from build123d import *

# Parameters (mm, degrees)
SKETCH1_W                    = 286
SKETCH1_H                    = 27
SKETCH1_R                    = 2
BOSS_EXTRUDE1_DEPTH          = 3
EDGE_FLANGE3_STRIP_W         = 13
EDGE_FLANGE3_STRIP_H         = 3
EDGE_FLANGE3_STRIP_CUT_DEPTH = 286
EDGE_FLANGE3_DEPTH           = 286


# Sheet-metal steps are written as plain solids
with BuildPart() as part:
    # Sketch1 → Boss-Extrude1 (new body)
    with BuildSketch(Plane(origin=(0, 0, 0), x_dir=(1, 0, 0), z_dir=(0, 1, 0))):
        with Locations((-143, 13.5)):
            Rectangle(SKETCH1_W, SKETCH1_H)
        with Locations(Location((-278, 21.5, 0), (0, 0, 270))):
            Circle(SKETCH1_R, mode=Mode.SUBTRACT)
        with Locations(Location((-278, 5.5, 0), (0, 0, 270))):
            Circle(SKETCH1_R, mode=Mode.SUBTRACT)
        with Locations(Location((-8, 21.5, 0), (0, 0, 90))):
            Circle(SKETCH1_R, mode=Mode.SUBTRACT)
        with Locations(Location((-8, 5.5, 0), (0, 0, 90))):
            Circle(SKETCH1_R, mode=Mode.SUBTRACT)
    extrude(amount=BOSS_EXTRUDE1_DEPTH)

    # Edge-Flange3 strip (across the edge) → Edge-Flange3 strip cut (cut)
    with BuildSketch(Plane(origin=(0, 3, -27), x_dir=(0, 0, 1), z_dir=(-1, 0, 0))):
        with Locations((-6, -1.5)):
            Rectangle(EDGE_FLANGE3_STRIP_W, EDGE_FLANGE3_STRIP_H)
    extrude(amount=EDGE_FLANGE3_STRIP_CUT_DEPTH, mode=Mode.SUBTRACT)

    # Edge-Flange3 section (across the edge) → Edge-Flange3 (add)
    with BuildSketch(Plane(origin=(0, 3, -27), x_dir=(0, 0, 1), z_dir=(-1, 0, 0))):
        with BuildLine():
            Line((-3, 0.5), (-3, 10))
            Line((-3, 10), (0, 10))
            Line((0, 10), (0, 0.5))
            ThreePointArc((0, 0.5), (0.146446609, 0.146446609), (0.5, 0))
            Line((0.5, 0), (0.5, -3))
            ThreePointArc((0.5, -3), (-1.974873734, -1.974873734), (-3, 0.5))
        make_face()
    extrude(amount=EDGE_FLANGE3_DEPTH)


solid = part.part
Here's how the part is built. I have some questions about the finished solid (model axes, mm). A direction names the side the tool comes from. Coordinates: 2 decimals unless noted, no trailing zeros. Order: outer loops, then holes, each group sorted by start corner. A loop starts at its lowest first (then second) coordinate and runs counter-clockwise, first axis right, second up. Notation, with made-up numbers: (79, 70) -> (116, 70) arc R16 cw to (116, 95) -> close; hole circle Ø9 at (-8.5, 6.25). An arc over 180 degrees is marked (long way). Answer in a Markdown table with one row per item.
(1) I want a section at C-C on z = -12. List the corners of the cut face in (x, y) for me, then the cut area to 3 significant figures.
Answer key:
| item | result |
|---|---|
| outline | (-286, 0) -> (0, 0) -> (0, 3) -> (-286, 3) -> close |
| area | 858 mm^2 |
(2) On a 3-axis mill with a long thin cutter (end or side, diameter ignored), from which of +Z, -Z, +X, -X, +Y, -Y can I reach the whole of each face in a straight line? I mean faces 1 (the face through (-145, 0, -13)), 2 (the face through (-141, 8, -27)). Say none if no direction works.
Answer key:
| item | result |
|---|---|
| face 1 | +Z, -Z, +X, -X, -Y |
| face 2 | +Z, +X, -X, +Y |
(3) I want a section at B-B on y = 7.75. List the corners of the cut face in (x, z) for me, then the cut area to 3 significant figures.
Answer key:
| item | result |
|---|---|
| outline | (-286, -30) -> (0, -30) -> (0, -27) -> (-286, -27) -> close |
| area | 858 mm^2 |
(4) Please list where these lines run through material, in increasing order: probe 1 along Z at (x, y) = (-8, 1.75); probe 2 along Z at (x, y) = (-8, 1.6); probe 3 along Y at (x, z) = (-261.5, -23.5).
Answer key:
| item | result |
|---|---|
| probe 1 | -29.53 to -23.5, -19.5 to -7.5, -3.5 to 0 |
| probe 2 | -29.44 to -23.5, -19.5 to -7.5, -3.5 to 0 |
| probe 3 | 0 to 3 |
(5) I want a section at A-A on x = -130. List the corners of the cut face in (y, z) for me, then the cut area to 3 significant figures.
Answer key:
| item | result |
|---|---|
| outline | (0, -26.5) arc R3.5 ccw to (3.5, -30) -> (13, -30) -> (13, -27) -> (3.5, -27) arc R0.5 cw to (3, -26.5) -> (3, 0) -> (0, 0) -> close |
| area | 117 mm^2 |
(6) Will these pins go through, and if not, where does the flat tip stop? pin 1 Ø3 at (x, z) = (-110.5, -7) entering from -Y; pin 2 Ø7.5 at (x, y) = (-129.5, 8.5) entering from +Z; pin 3 Ø2 at (x, z) = (-156, -24) entering from +Y.
Answer key:
| item | result |
|---|---|
| pin 1 | y = 0 |
| pin 2 | z = -27 |
| pin 3 | y = 3 |
